from build123d import *

# Parameters (mm, degrees)
F1_DEPTH = 152.4
F3_DEPTH = 6.35
F5_DEPTH = 6.35
F7_DEPTH = 101.6


with BuildPart() as f1:
    # F0 (on Front) → F1 (new body)
    with BuildSketch(Plane.XZ):
        Polygon((-3.6661742094, -6.35), (3.6661742094, -6.35), (7.3323484187, 0), (3.6661742094, 6.35), (-3.6661742094, 6.35), (-7.3323484187, 0), align=None)
    extrude(amount=F1_DEPTH)

    # F2 (on face) → F3 (join)
    with BuildSketch(Plane.XZ.offset(152.4)):
        with BuildLine():
            ThreePointArc((5.499261351, -3.174999936), (6.1336290065, -1.6435009007), (6.35, 0))
            ThreePointArc((6.35, 0), (6.133629012, 1.6435008802), (5.4992613723, 3.1749998991))
            ThreePointArc((5.4992613723, 3.1749998991), (3.1750000504, 5.4992612849), (0, 6.35))
            ThreePointArc((0, 6.35), (-3.1749999838, 5.4992613234), (-5.4992612953, 3.1750000324))
            ThreePointArc((-5.4992612953, 3.1750000324), (-6.35, 2.13e-08), (-5.4992613166, -3.1749999956))
            ThreePointArc((-5.4992613166, -3.1749999956), (-3.1750000022, -5.4992613128), (0, -6.35))
            ThreePointArc((0, -6.35), (3.175000032, -5.4992612955), (5.499261351, -3.174999936))
        make_face()
    extrude(amount=F3_DEPTH)

    # F4 (on face) → F5 (join)
    with BuildSketch(Plane(origin=(0, 0, 0), x_dir=(-1, 0, 0), z_dir=(0, 1, 0))):
        with BuildLine():
            ThreePointArc((5.4992613166, -3.1749999956), (6.1336289976, -1.6435009339), (6.35, 0))
            ThreePointArc((6.35, 0), (6.1336289972, 1.6435009354), (5.499261315, 3.1749999983))
            ThreePointArc((5.499261315, 3.1749999983), (3.1750000009, 5.4992613135), (0, 6.35))
            ThreePointArc((0, 6.35), (-3.174999954, 5.4992613406), (-5.4992612609, 3.175000092))
            ThreePointArc((-5.4992612609, 3.175000092), (-6.35, 7.29e-08), (-5.4992613338, -3.1749999658))
            ThreePointArc((-5.4992613338, -3.1749999658), (-3.1750000171, -5.4992613042), (0, -6.35))
            ThreePointArc((0, -6.35), (3.1750000022, -5.4992613128), (5.4992613166, -3.1749999956))
        make_face()
    extrude(amount=F5_DEPTH)

    # F6 (on face) → F7 (join)
    with BuildSketch(Plane(origin=(0, 6.35, 0), x_dir=(-1, 0, 0), z_dir=(0, 1, 0))):
        with BuildLine():
            ThreePointArc((-5.4992611496, -3.1750002849), (-3.1749998554, -5.4992613975), (5e-09, -6.35))
            ThreePointArc((5e-09, -6.35), (3.174999908, -5.4992613672), (5.4992612052, -3.1750001884))
            ThreePointArc((5.4992612052, -3.1750001884), (6.1336289688, -1.6435010415), (6.35, 0))
            ThreePointArc((6.35, 0), (6.1336289832, 1.6435009877), (5.4992612609, 3.175000092))
            ThreePointArc((5.4992612609, 3.175000092), (3.174999954, 5.4992613406), (0, 6.35))
            ThreePointArc((0, 6.35), (-3.1750000802, 5.4992612677), (-5.4992614067, 3.1749998395))
            ThreePointArc((-5.4992614067, 3.1749998395), (-6.35, -2.571e-07), (-5.4992611496, -3.1750002849))
        make_face()
        with BuildLine():
            Line((5e-09, -6.35), (3.6661742094, -6.35))
            Line((3.6661742094, -6.35), (5.4992612052, -3.1750001884))
            ThreePointArc((5.4992612052, -3.1750001884), (3.174999908, -5.4992613672), (5e-09, -6.35))
        make_face()
        with BuildLine():
            ThreePointArc((6.35, 0), (6.1336289688, -1.6435010415), (5.4992612052, -3.1750001884))
            Line((5.4992612052, -3.1750001884), (7.3323484187, 0))
            Line((7.3323484187, 0), (5.4992612609, 3.175000092))
            ThreePointArc((5.4992612609, 3.175000092), (6.1336289832, 1.6435009877), (6.35, 0))
        make_face()
        with BuildLine():
            ThreePointArc((0, 6.35), (3.174999954, 5.4992613406), (5.4992612609, 3.175000092))
            Line((5.4992612609, 3.175000092), (3.6661742094, 6.35))
            Line((3.6661742094, 6.35), (0, 6.35))
        make_face()
        with BuildLine():
            Line((-3.6661742094, 6.35), (-5.4992614067, 3.1749998395))
            ThreePointArc((-5.4992614067, 3.1749998395), (-3.1750000802, 5.4992612677), (0, 6.35))
            Line((0, 6.35), (-3.6661742094, 6.35))
        make_face()
        with BuildLine():
            Line((-7.3323484187, 0), (-5.4992611496, -3.1750002849))
            ThreePointArc((-5.4992611496, -3.1750002849), (-6.35, -2.571e-07), (-5.4992614067, 3.1749998395))
            Line((-5.4992614067, 3.1749998395), (-7.3323484187, 0))
        make_face()
        with BuildLine():
            Line((-3.6661742094, -6.35), (5e-09, -6.35))
            ThreePointArc((5e-09, -6.35), (-3.1749998554, -5.4992613975), (-5.4992611496, -3.1750002849))
            Line((-5.4992611496, -3.1750002849), (-3.6661742094, -6.35))
        make_face()
    extrude(amount=F7_DEPTH)


solid = f1.part
Here's how the part is built. I have some questions about the finished solid (model axes, mm). Coordinates: 2 decimals unless noted, no trailing zeros. Order: outer loops, then holes, each group sorted by start corner. A loop starts at its lowest first (then second) coordinate and runs counter-clockwise, first axis right, second up.
Item 1: If we section it at A-A on y = -39: List the corners of the cut face in (x, z) for me.
Result sheet:
outline: (-7.33, 0) - (-3.67, -6.35) - (3.67, -6.35) - (7.33, 0) - (3.67, 6.35) - (-3.67, 6.35) - close
Item 2: I need wall thicknesses on line 1 (X direction, y = -37, z = 1.75); line 2 (Z direction, x = -5.5, y = -67); line 3 (X direction, y = -129.5, z = 1) (3 decimals). Which ranges of each line are inside material? Lowest first, please.
Result sheet:
line 1: x = -6.32 to 6.32
line 2: z = -3.17 to 3.17
line 3: x = -6.755 to 6.755
Item 3: For P1, Ø6, axis at x = 5.5, y = -94, coming from the +Z side; P2, Ø6, axis at y = -74, z = -4, coming from the +X side (3 decimals); P3, Ø3, axis at y = -33, z = -4, coming from the +X side; P4, Ø2, axis at y = -13.5, z = 5, coming from the +X side, each with a flat end and sliding along its axis, tell me the tip position at first contact or that it passes through.
Result sheet:
P1: stops at z = 6.35
P2: stops at x = 6.755
P3: stops at x = 5.89
P4: stops at x = 5.02
